from build123d import *

# Parameters (mm, degrees)
SKETCH_R                 = 3.05
PAD_DEPTH                = 7
PAD_DEPTH_BACK           = 10
SKETCH001_R              = 1.05
POCKET_DEPTH             = 5
FILLET_R                 = 0.5
CLONE001_PLACEMENT_ANGLE = 90


with BuildPart() as part:
    # Sketch → Pad (new body, two sides)
    with BuildSketch(Plane.XZ) as pad_sk:
        with BuildLine():
            Line((10, 0), (10, -5))
            Line((10, -5), (-10, -5))
            Line((-10, -5), (-10, 0))
            Line((-10, 0), (-5, 0))
            ThreePointArc((5, 0), (0, 5), (-5, 0))
            Line((10, 0), (5, 0))
        make_face()
        Circle(SKETCH_R, mode=Mode.SUBTRACT)
    extrude(amount=PAD_DEPTH)
    extrude(pad_sk.sketch, amount=-PAD_DEPTH_BACK)

    # Sketch001 → Pocket (cut)
    with BuildSketch(Plane(origin=(0, 0, -5), x_dir=(1, 0, 0), z_dir=(0, 0, -1))):
        with Locations((-7.5, 4.5)):
            Circle(SKETCH001_R)
        with Locations((-7.5, -7.5)):
            Circle(SKETCH001_R)
        with Locations((7.5, -7.5)):
            Circle(SKETCH001_R)
        with Locations((7.5, 4.5)):
            Circle(SKETCH001_R)
    extrude(amount=-POCKET_DEPTH, mode=Mode.SUBTRACT)

    # Fillet
    fillet_edges = [part.edges().sort_by_distance(p)[0] for p in [
        (-3.05, 10, 0),
        (-3.05, -7, 0),
    ]]
    fillet(fillet_edges, radius=FILLET_R)


with BuildPart() as part_1:
    # Clone001 placement: moved
    add(part.part.moved(Location((44, -105, 11))).rotate(Axis((44, -105, 11), (0, 0, 1)), CLONE001_PLACEMENT_ANGLE))


solid = part_1.part
Verification items for the finished model (mm, model axes). A direction names the side the tool comes from. Coordinates: 2 decimals unless noted, no trailing zeros. Loops run counter-clockwise (first coordinate to the right, second up) from the corner with the lowest first, then second, coordinate; pieces in that order, holes last. Notation, with made-up numbers: M 20,42 L 72,42 A17 ccw 72,64 Z; hole C 25.5,-3.75 d7. An arc over 180 degrees is marked long. One line per item, written item: value.
1. Section check C-C on x = 44.5. Record the cut outline in (y, z), plus the area to 3 significant figures.
Answers follow:
outline: M -115,6 L -95,6 L -95,11 L -100,11 A5 ccw -110,11 L -115,11 Z; hole C -105,11 d6.1
area: 110 mm^2
2. Material ranges on line 1 along X through (y, z) = (-97.5, 8.1); line 2 along Z through (x, y) = (40.5, -105); line 3 along Z through (x, y) = (44, -107.75), recorded low to high. Write a range as from..to.
Answers follow:
line 1: 34..35.45, 37.55..47.45, 49.55..51
line 2: 6..7.95, 14.05..16
line 3: 6..9.68, 12.32..15.18
3. Mould release check, pull along Y, two halves, no side actions. Record for faces 1 (the flat face through (43, -115, 8)), 2 (the cylindrical face through (43, -105, 16)), 3 (the cylindrical face through (48.1, -96.53, 8.46)): pulls with the +Y half, pulls with the -Y half, needs draft (parallel to the pull), parting line crosses it, or undercut.
Answers follow:
face 1: pulls with the -Y half
face 2: parting line crosses it
face 3: undercut
4. Section check B-B on y = -97.5. Record the cut outline in (x, z), plus the area to 3 significant figures.
Answers follow:
outline: M 34,6 L 35.45,6 L 35.45,11 L 34,11 Z; M 37.55,6 L 47.45,6 L 47.45,11 L 37.55,11 Z; M 49.55,6 L 51,6 L 51,11 L 49.55,11 Z
area: 64.0 mm^2
5. Set-up check for faces 4 (the flat face through (43, -113, 11)), 5 (the flat face through (43, -97, 11)), 6 (the flat face through (51, -107.1, 7.7)): record each of +Z, -Z, +X, -X, +Y, -Y from which the full face is reachable in a straight line by a thin tool's end or side.
Answers follow:
face 4: +Z, +X, -X, -Y
face 5: +Z, +X, -X, +Y
face 6: +Z, -Z, +X, +Y, -Y
6. Section check A-A on x = 48.5. Record the cut outline in (y, z), plus the area to 3 significant figures.
Answers follow:
outline: M -115,6 L -113.55,6 L -113.55,11 L -115,11 Z; M -111.45,6 L -98.55,6 L -98.55,11 L -100,11 A5 ccw -110,11 L -111.45,11 Z; M -96.45,6 L -95,6 L -95,11 L -96.45,11 Z; hole C -105,11 d6.1
area: 89.0 mm^2
7. Section check D-D on z = 9.75. Give the number of separate pieces and of enclosed holes in the cut face, plus the area to 3 significant figures.
Answers follow:
separate pieces: 2
enclosed holes: 4
area: 231 mm^2
8. Gauge pin test, flat ends, axial feed: P1, Ø5.5, axis at x = 39, y = -113.5, coming from the +Z side; P2, Ø8, axis at x = 39.5, y = -113, coming from the +Z side. Record the tip position at first contact, or that the pin passes through.
Answers follow:
P1: z = 11
P2: z = 14
